from build123d import *

# Parameters (mm, degrees)
BOSS_EXTRUDE1_DEPTH = 130.175


with BuildPart() as part:
    # Sketch1 → Boss-Extrude1 (new body)
    with BuildSketch(Plane(origin=(0, 0, 0), x_dir=(0, 0, -1), z_dir=(1, 0, 0))):
        with BuildLine():
            Line((176.178529946, -50.8), (177.830117427, -50.8))
            ThreePointArc((177.830117427, -50.8), (182.392106967, 30.615518615), (151.497050891, 106.07937705))
            Line((151.497050891, 106.07937705), (150.196647021, 105.168824458))
            ThreePointArc((150.196647021, 105.168824458), (174.869963651, 55.13628775), (183.35625, 0))
            ThreePointArc((183.35625, 0), (181.552952325, -25.652288715), (176.178529946, -50.8))
        make_face()
    extrude(amount=BOSS_EXTRUDE1_DEPTH)


solid = part.part
Check sheet for the modelled part. Datum: model origin and axes. Units: mm. Round coordinates to 2 decimals unless told otherwise and drop trailing zeros. Loops run counter-clockwise (first coordinate to the right, second up) from the corner with the lowest first, then second, coordinate; pieces in that order, holes last. Notation, with made-up numbers: M -14.75,38.5 L 32.25,38.5 A34 ccw 32.25,71.5 Z; hole C 78.25,5.25 d1. An arc over 180 degrees is marked long. One line per item, written item: value.
(1) Sectioned sample at C-C, the plane z = -172.5. Record the cut outline in (x, y) (3 decimals), then the cut area to 3 significant figures.
Computed values:
outline: M 0,62.155 L 130.175,62.155 L 130.175,66.693 L 0,66.693 Z
area: 591 mm^2
(2) Sectioned sample at B-B, the plane y = 54.5. Record the cut outline in (x, z) (3 decimals), then the cut area to 3 significant figures.
Computed values:
outline: M 0,-176.731 L 130.175,-176.731 L 130.175,-175.069 L 0,-175.069 Z
area: 216 mm^2
(3) Sectioned sample at A-A, the plane x = 17. Record the cut outline in (y, z), then the cut area to 3 significant figures.
Computed values:
outline: M -50.8,-177.83 A184.94 ccw 106.08,-151.5 L 105.17,-150.2 A183.36 cw -50.8,-176.18 Z
area: 260 mm^2
(4) Thickness scan on line 1 (Z direction, x = 9, y = 0.5); line 2 (Y direction, x = 71, z = -155); line 3 (Z direction, x = 105.5, y = -21.5). Record the ranges inside material, lowest first.
Computed values:
line 1: z = -184.94 to -183.36
line 2: y = 97.95 to 100.89
line 3: z = -183.69 to -182.09
(5) Depth check by flat-ended pin: pin 1 Ø3 at (x, y) = (29, -17) entering from +Z; pin 2 Ø6 at (x, z) = (98.5, -163.5) entering from -Y. Enter the tip coordinate at first touch or a pass-through.
Computed values:
pin 1: stops at z = -182.42
pin 2: stops at y = 76.79
